Geometry: final body of the model. Coordinates: model frame, mm. A direction names the side the tool comes from. Give positions to 0.01 mm unless a question says otherwise; leave off trailing zeros. Write each loop counter-clockwise with the first axis right and the second up, starting at its lowest first coordinate (ties: lowest second). Pieces come first, ordered by that corner, then holes.
```python
from build123d import *

# Parameters (mm, degrees)
F0_W       = 48
F0_H       = 20
F1_DEPTH   = 3
F2_W       = 30
F2_H       = 1.5
F3_DEPTH   = 15
F6_D       = 3
F6_ON_F5_D = 3
F7_W       = 30
F7_H       = 15
F8_DEPTH   = 2.5
F11_DEPTH  = 1
F12_DEPTH  = 1


with BuildPart() as f1:
    # F0 (on Top) → F1 (new body)
    with BuildSketch(Plane.XY):
        Rectangle(F0_W, F0_H)
    extrude(amount=F1_DEPTH)

    # F2 (on face) → F3 (join)
    with BuildSketch(Plane.XY.offset(3)):
        with Locations((-9, -9.25)):
            Rectangle(F2_W, F2_H)
    extrude(amount=F3_DEPTH)

    # F6 (through all)
    with Locations(Plane.XZ.offset(10)):
        with Locations((0, 10.5), (-18, 10.5)):
            Hole(F6_D / 2)

    # F6 on F5 (through all)
    with Locations(Plane.XY.offset(3)):
        with Locations((19, 5), (12, 5), (12, -5)):
            Hole(F6_ON_F5_D / 2)

    # F7 (on face) → F8 (join)
    with BuildSketch(Plane(origin=(0, -8.5, 0), x_dir=(-1, 0, 0), z_dir=(0, 1, 0))):
        with Locations((9, 10.5)):
            Rectangle(F7_W, F7_H)
        Polygon((2.4, 11.8856406461), (2.4, 9.1143593539), (0, 7.7287187079), (-2.4, 9.1143593539), (-2.4, 11.8856406461), (0, 13.2712812921), align=None, mode=Mode.SUBTRACT)
        Polygon((20.4, 9.1143593539), (18, 7.7287187079), (15.6, 9.1143593539), (15.6, 11.8856406461), (18, 13.2712812921), (20.4, 11.8856406461), align=None, mode=Mode.SUBTRACT)
    extrude(amount=F8_DEPTH)

    # F9 (on face) → F11 (join)
    with BuildSketch(Plane(origin=(-24, 0, 0), x_dir=(0, -1, 0), z_dir=(-1, 0, 0))):
        Polygon((6, 18), (-10, 3), (6, 3), align=None)
    extrude(amount=-F11_DEPTH)

    # F10 (on face) → F12 (join)
    with BuildSketch(Plane.YZ.offset(6)):
        Polygon((10, 3), (-6, 18), (-6, 3), align=None)
    extrude(amount=-F12_DEPTH)


solid = f1.part
```
Item 1: Line query: L1, parallel to Y at x = 12, z = 0.8; L2, parallel to X at y = -1, z = 5.5; L3, parallel to Y at x = -3.5, z = 8. Output: solid intervals per line, ascending.
Found:
L1: y = -10 to -6.5, -3.5 to 3.5, 6.5 to 10
L2: x = -24 to -23, 5 to 6
L3: y = -10 to -6
Item 2: Section B-B, the plane x = 19. Return the cut outline in (y, z), plus the area to 3 significant figures.
Found:
outline: (-10, 0) - (3.5, 0) - (3.5, 3) - (-10, 3) - close; (6.5, 0) - (10, 0) - (10, 3) - (6.5, 3) - close
area: 51.0 mm2
Item 3: Section C-C, the plane y = 5. Return the cut outline in (x, z), plus the area to 3 significant figures.
Found:
outline: (-24, 0) - (10.5, 0) - (10.5, 3) - (6, 3) - (6, 7.69) - (5, 7.69) - (5, 3) - (-23, 3) - (-23, 7.69) - (-24, 7.69) - close; (13.5, 0) - (17.5, 0) - (17.5, 3) - (13.5, 3) - close; (20.5, 0) - (24, 0) - (24, 3) - (20.5, 3) - close
area: 135 mm2
Item 4: Reachability of faces 1 (the face through (-9, -6, 11)), 2 (the face through (-1.18, -7.27, 12.59)), 3 (the face through (15, 0, 3)), 4 (the face through (24, 0, 1)) from +Z, -Z, +X, -X, +Y, -Y: full face, straight path, thin tool, end or side. Return the list, or none.
Found:
face 1: +Z, +Y
face 2: +Y
face 3: +Z, +X, +Y, -Y
face 4: +Z, -Z, +X, +Y, -Y
Item 5: Pull-direction query (Z, two-part tool) for faces 5 (the face through (0, -9, 9)), 6 (the face through (-6, -10, 9)), 7 (the face through (-23.507, 1.888, 10.605)); classes: +Z half, -Z half, draft (parallel to the pull), parting line (faces both ways), or undercut.
Found:
face 5: undercut
face 6: draft
face 7: +Z half
Item 6: Section A-A, the plane z = 10.5. Return the cut outline in (x, y).
Found:
outline: (-24, -10) - (-19.5, -10) - (-19.5, -8.5) - (-20.4, -8.5) - (-20.4, -6) - (-23, -6) - (-23, 2) - (-24, 2) - close; (-16.5, -10) - (-1.5, -10) - (-1.5, -8.5) - (-2.4, -8.5) - (-2.4, -6) - (-15.6, -6) - (-15.6, -8.5) - (-16.5, -8.5) - close; (1.5, -10) - (6, -10) - (6, 2) - (5, 2) - (5, -6) - (2.4, -6) - (2.4, -8.5) - (1.5, -8.5) - close
Item 7: Section D-D, the plane x = 12. Return the cut outline in (y, z).
Found:
outline: (-10, 0) - (-6.5, 0) - (-6.5, 3) - (-10, 3) - close; (-3.5, 0) - (3.5, 0) - (3.5, 3) - (-3.5, 3) - close; (6.5, 0) - (10, 0) - (10, 3) - (6.5, 3) - close
Item 8: Pin query (flat end, axial travel): pin 1 Ø4 at (y, z) = (-1.5, 9) entering from +X; pin 2 Ø5.5 at (x, y) = (15.5, -5) entering from +Z; pin 3 Ø2.5 at (x, y) = (12, 5) entering from -Z; pin 4 Ø4.5 at (x, z) = (-13.5, 14) entering from +Y. Return the tip coordinate at first contact, or that it passes through.
Found:
pin 1: stops at x = 6
pin 2: stops at z = 3
pin 3: passes through
pin 4: stops at y = -6
